Input: part model. Units: mm. Frame: model coordinates. A direction names the side the tool comes from. Give positions to 0.01 mm unless a question says otherwise; leave off trailing zeros. Loops run counter-clockwise (first coordinate to the right, second up) from the corner with the lowest first, then second, coordinate; pieces in that order, holes last. Notation, with made-up numbers: (66, -21.75) - (116, -21.75) arc R35 cw to (116, 15.25) - close; hole circle Ø7 at (36.5, -9). An arc over 180 degrees is marked (long way). Answer as a JSON object with one key per item and string values.
from build123d import *

# Parameters (mm, degrees)
SKETCH1_W           = 35
SKETCH1_H           = 8.75
BOSS_EXTRUDE1_DEPTH = 20
SKETCH2_R           = 3.5
BOSS_EXTRUDE2_DEPTH = 2
SKETCH3_R           = 1.5
CUT_EXTRUDE1_DEPTH  = 2
FILLET1_R           = 2


with BuildPart() as part:
    # Sketch1 → Boss-Extrude1 (new body)
    with BuildSketch(Plane(origin=(0, 0, 0), x_dir=(1, 0, 0), z_dir=(0, 1, 0))):
        Rectangle(SKETCH1_W, SKETCH1_H)
    extrude(amount=BOSS_EXTRUDE1_DEPTH)

    # Sketch2 → Boss-Extrude2 (add)
    with BuildSketch(Plane(origin=(17.5, 0, 0), x_dir=(0, 0, -1), z_dir=(1, 0, 0))):
        with Locations(Location((0, 16, 0), (0, 0, 180))):
            Circle(SKETCH2_R)
    extrude(amount=BOSS_EXTRUDE2_DEPTH)

    # Sketch3 → Cut-Extrude1 (cut)
    with BuildSketch(Plane(origin=(19.5, 0, 0), x_dir=(0, 0, -1), z_dir=(1, 0, 0))):
        with Locations((0, 16)):
            Circle(SKETCH3_R)
    extrude(amount=-CUT_EXTRUDE1_DEPTH, mode=Mode.SUBTRACT)

    # Fillet1
    fillet1_edges = [part.edges().sort_by_distance(p)[0] for p in [
        (19.5, 16, -3.5),
    ]]
    fillet(fillet1_edges, radius=FILLET1_R - 0.0001)  # a hair under: the kernel refuses the full size


solid = part.part
Item 1: Access query for faces 1 (the face through (18.51, 17.01, 1.11)), 2 (the face through (-17.5, 10, 0)). Directions: +Z, -Z, +X, -X, +Y, -Y. A direction counts if a zero-diameter tool reaches every point of the face in a straight line with its end or side. Return the directions, or none.
Geometry check:
{"face 1": "+X", "face 2": "+Z, -Z, -X, +Y, -Y"}
Item 2: Material intervals for line 1 (X direction, y = 4.75, z = -1.5); line 2 (Y direction, x = 18.65, z = 0); line 3 (Y direction, x = 18.95, z = 0), sorted ascending. Write a range as [from, to].
Geometry check:
{"line 1": "x = [-17.5, 17.5]", "line 2": "y = [12.86, 14.5], [17.5, 19.14]", "line 3": "y = [13.12, 14.5], [17.5, 18.88]"}
Item 3: Mould query, pull axis Z, two halves, no side actions, for faces 3 (the face through (0, 0, 0)), 4 (the face through (17.5, 16, 0)), 5 (the face through (0, 10, -4.375)). Classes: released by +Z, released by -Z, zero draft, split by the parting line, or undercut.
Geometry check:
{"face 3": "zero draft", "face 4": "undercut", "face 5": "released by -Z"}
Item 4: Cut plane A-A (y = 12). Return loops of the section in (x, z) (3 decimals).
Geometry check:
{"outline": "(-17.5, -4.375) - (17.5, -4.375) - (17.5, 4.375) - (-17.5, 4.375) - close"}
Item 5: Contact query for a flat-ended pin moving along its axis: P1, Ø4.5, axis at y = 9.5, z = 1.5, coming from the +X side. Output: stop coordinate, or through.
Geometry check:
{"P1": "stops at x = 17.5"}
